Source: CAD feature listing. Evaluate the final solid. Frame: model axes, mm. A direction names the side the tool comes from. Round coordinates to 2 decimals unless told otherwise and drop trailing zeros. Write each loop counter-clockwise with the first axis right and the second up, starting at its lowest first coordinate (ties: lowest second). Pieces come first, ordered by that corner, then holes.
```python
from build123d import *

# Parameters (mm, degrees)
ESQUISSE1_R        = 2.5
BOSS_EXTRU_1_DEPTH = 5


with BuildPart() as part:
    # Esquisse1 → Boss.-Extru.1 (new body)
    with BuildSketch(Plane(origin=(0, 0, 0), x_dir=(1, 0, 0), z_dir=(0, 1, 0))):
        with BuildLine():
            Line((30.416462038, 3.875687745), (55.823272708, -6.059403674))
            ThreePointArc((55.823272708, -6.059403674), (73.630583756, -4.03622534), (82, 11.811375395))
            Line((82, 11.811375395), (82, 110.123102525))
            Line((82, 110.123102525), (109.832159843, 110.123102525))
            Line((109.832159843, 110.123102525), (109.832159843, 119.415014129))
            Line((109.832159843, 119.415014129), (41.252434476, 119.415014129))
            Line((41.252434476, 119.415014129), (41.252434476, 110.123102525))
            Line((41.252434476, 110.123102525), (62, 110.123102525))
            Line((62, 110.123102525), (62, 13))
            Line((62, 13), (38.173084143, 22.317288594))
            ThreePointArc((38.173084143, 22.317288594), (11.245695012, 22.487512145), (-8.882082163, 4.599363906))
            ThreePointArc((-8.882082163, 4.599363906), (-4.515728742, -8.924893603), (8.966917542, -4.431695127))
            ThreePointArc((8.966917542, -4.431695127), (18.075204101, 3.89573938), (30.416462038, 3.875687745))
        make_face()
        Circle(ESQUISSE1_R, mode=Mode.SUBTRACT)
    extrude(amount=BOSS_EXTRU_1_DEPTH)


solid = part.part
```
Q1. Section query A-A, the plane x = 0. Output: boundary loops of the cut face in (y, z), and give its area (3 significant figures).
Q2. Mould query, pull axis X, two halves, no side actions, for faces 5 (the face through (82, 2, -60)), 6 (the face through (42.94, 2.46, 1.02)), 7 (the face through (76, 2, -119.415)). Classes: pulls with the +X half, pulls with the -X half, needs draft (parallel to the pull), parting line crosses it, or undercut.
Q3. Set-up query: faces 1 (the face through (41.252, 2, -115)), 2 (the face through (51, 2, -110.123)), 3 (the face through (50.253, 2.465, -17.593)), 4 (the face through (96, 2, -110.123)). Return all of +Z, -Z, +X, -X, +Y, -Y with unobstructed straight access to the full face (end or side cutting, diameter ignored); none if empty.
Q4. Section query D-D, the plane z = -58.5. Output: boundary loops of the cut face in (x, y), and give its area (3 significant figures).
Q5. Section query B-B, the plane y = 2.5. Output: boundary loops of the cut face in (x, z), and give its area (3 significant figures).
Q6. Pin query (flat end, axial travel): P1, Ø2.5, axis at y = 1.5, z = -78.5, coming from the -X side; P2, Ø4, axis at x = 0, z = 0, coming from the +Y side; P3, Ø1.5, axis at x = 39, y = 0.5, coming from the +Z side; P4, Ø3, axis at x = 18.5, y = 0.5, coming from the -Z side. Return the tip coordinate at first contact, or that it passes through.
Q7. Line query: line 1 (X direction, y = 1.45, z = -70); line 2 (X direction, y = 2.9, z = -111); line 3 (Z direction, x = 0, y = 1.05). Output: solid intervals per line, ascending.
Q8. Section query C-C, the plane z = 0. Output: boundary loops of the cut face in (x, y).
Filled in:
1. outline: (0, -15.82) - (5, -15.82) - (5, -2.5) - (0, -2.5) - close; (0, 2.5) - (5, 2.5) - (5, 10) - (0, 10) - close
1. area: 104 mm2
2. face 5: pulls with the +X half
2. face 6: undercut
2. face 7: needs draft
3. face 1: -Z, -X, +Y, -Y
3. face 2: -X, +Y, -Y
3. face 3: +Y, -Y
3. face 4: +Z, +X, +Y, -Y
4. outline: (62, 0) - (82, 0) - (82, 5) - (62, 5) - close
4. area: 100 mm2
5. outline: (-8.88, -4.6) arc R37.58 ccw to (38.17, -22.32) - (62, -13) - (62, -110.12) - (41.25, -110.12) - (41.25, -119.42) - (109.83, -119.42) - (109.83, -110.12) - (82, -110.12) - (82, -11.81) arc R19.19 ccw to (55.82, 6.06) - (30.42, -3.88) arc R17.01 cw to (8.97, 4.43) arc R10 ccw (long way) to start; hole circle Ø5 at (0, 0)
5. area: 4,440 mm2
6. P1: stops at x = 62
6. P2: passes through
6. P3: stops at z = -0.23
6. P4: stops at z = -24.63
7. line 1: x = 62 to 82
7. line 2: x = 41.25 to 109.83
7. line 3: z = -15.82 to -2.5, 2.5 to 10
8. outline: (-10, 0) - (-2.5, 0) - (-2.5, 5) - (-10, 5) - close; (2.5, 0) - (12.13, 0) - (12.13, 5) - (2.5, 5) - close; (40.33, 0) - (77.93, 0) - (77.93, 5) - (40.33, 5) - close
